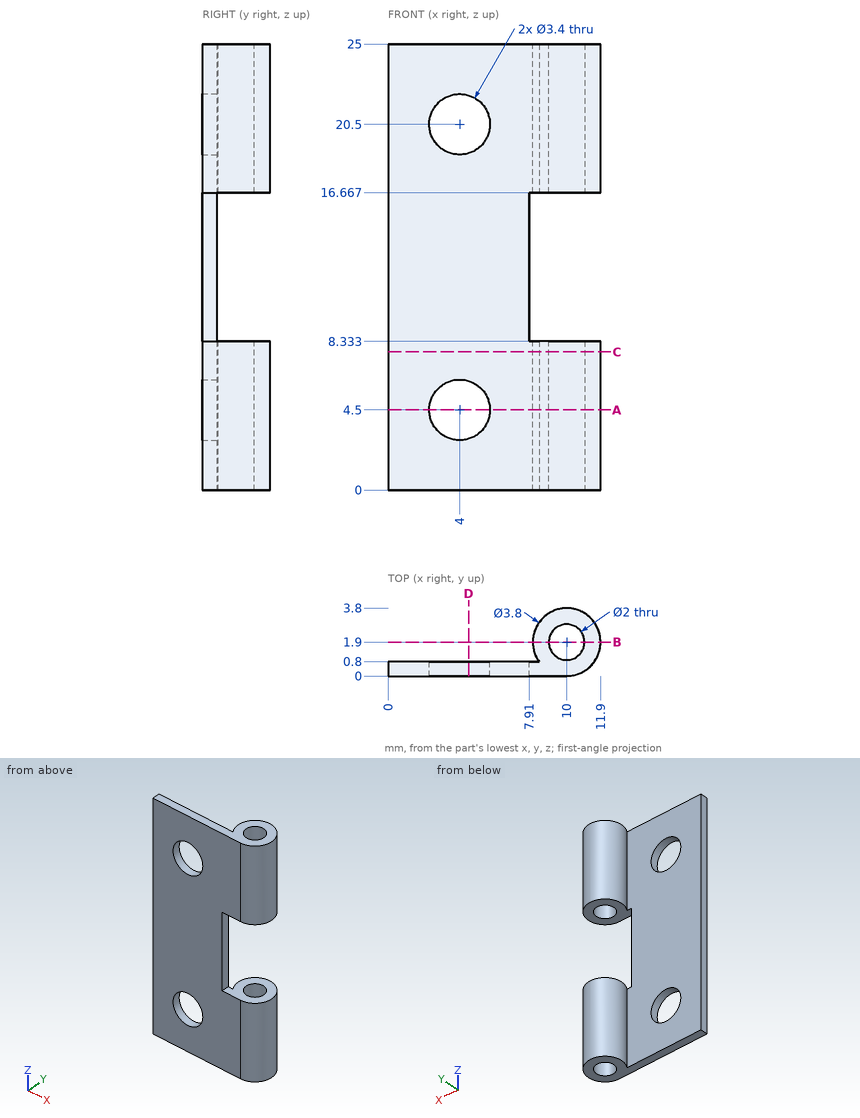
Print and shaded views of the part. All mm, measured from the part's lowest x, y and z. Give positions to 0.01 mm unless a question says otherwise; leave off trailing zeros. Loops run counter-clockwise (first coordinate to the right, second up) from the corner with the lowest first, then second, coordinate; pieces in that order, holes last. Notation, with made-up numbers: M 33,52 L 60,52 A10 ccw 60,66 Z; hole C 39,-28.5 d5. An arc over 180 degrees is marked long. Write each question's results on one line, items separated by ' | '.
Q1. Probe probe 1 along Z at (x, y) = (4, 0.45); probe 2 along Z at (x, y) = (11.25, 1.65); probe 3 along Y at (x, z) = (1.5, 6). List the from-to ranges inside material, lowest first.
Geometry check:
probe 1: z = 0 to 2.8, 6.2 to 18.8, 22.2 to 25 | probe 2: z = 0 to 8.33, 16.67 to 25 | probe 3: y = 0 to 0.8
Q2. Flat gauge pin, fed straight in: P1, Ø5.5, axis at x = 4, z = 20.5, coming from the +Y side. Where does the tip first touch, or does it go through?
Geometry check:
P1: stops at y = 0.8
Q3. Band-saw the part on B-B on y = 1.9. Write the cut outline in (x, z), and give its area (3 significant figures).
Geometry check:
outline: M 8.1,0 L 9,0 L 9,8.33 L 8.1,8.33 Z; M 8.1,16.67 L 9,16.67 L 9,25 L 8.1,25 Z; M 11,0 L 11.9,0 L 11.9,8.33 L 11,8.33 Z; M 11,16.67 L 11.9,16.67 L 11.9,25 L 11,25 Z | area: 30.0 mm²
Q4. Band-saw the part on D-D on x = 4.5. Write the cut outline in (y, z) (1 decimal), and give its area (3 significant figures).
Geometry check:
outline: M 0,0 L 0.8,0 L 0.8,2.9 L 0,2.9 Z; M 0,6.1 L 0.8,6.1 L 0.8,18.9 L 0,18.9 Z; M 0,22.1 L 0.8,22.1 L 0.8,25 L 0,25 Z | area: 14.8 mm²
Q5. Band-saw the part on C-C on z = 7.75. Write the cut outline in (x, y).
Geometry check:
outline: M 0,0 L 10,0 A1.9 ccw long 8.45,0.8 L 0,0.8 Z; hole C 10,1.9 d2
Q6. Band-saw the part on A-A on z = 4.5. Write the cut outline in (x, y).
Geometry check:
outline: M 0,0 L 2.3,0 L 2.3,0.8 L 0,0.8 Z; M 5.7,0 L 10,0 A1.9 ccw long 8.45,0.8 L 5.7,0.8 Z; hole C 10,1.9 d2
